The figure shows three views and two pictorial views of one solid part (mm, origin at its lowest corner). Answer the questions. A direction names the side the tool comes from. Coordinates: 2 decimals unless noted, no trailing zeros. Order: outer loops, then holes, each group sorted by start corner. A loop starts at its lowest first (then second) coordinate and runs counter-clockwise, first axis right, second up. Notation, with made-up numbers: (-6, 34.5) - (52, 34.5) arc R23 cw to (52, 70.5) - close; hole circle Ø4 at (-10.75, 74). An arc over 180 degrees is marked (long way). Answer as a JSON object with one key per item and string values. Group by question number.
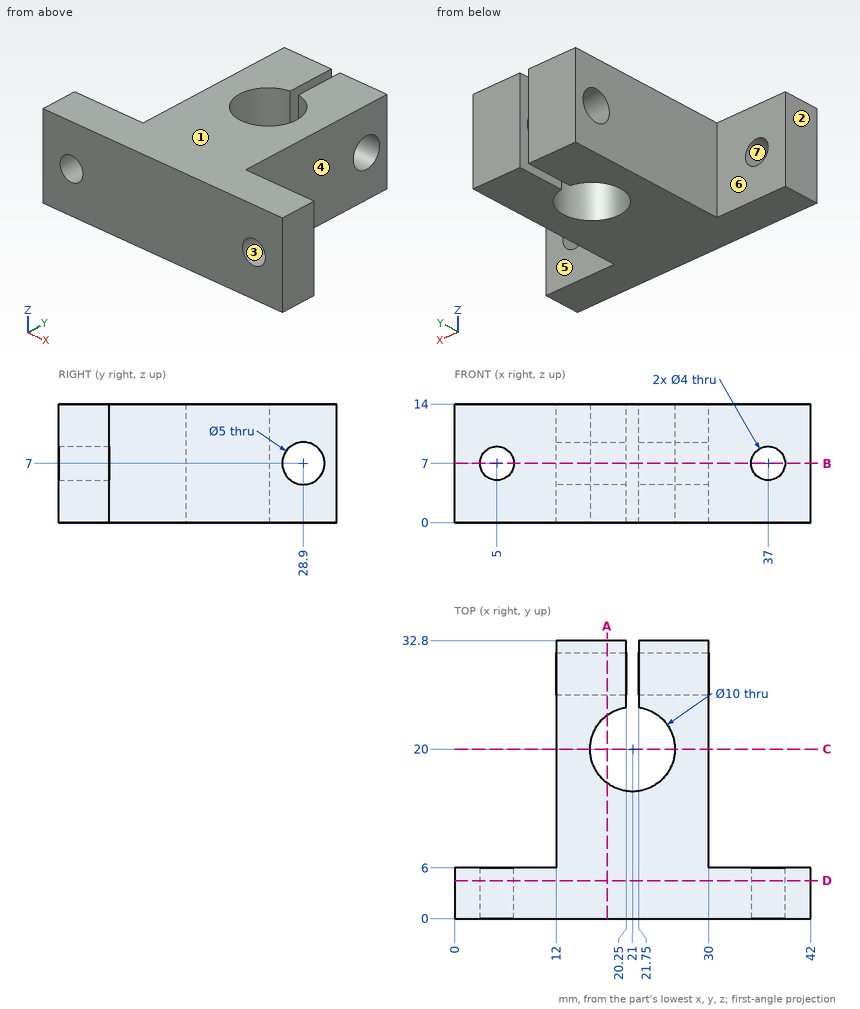
1. A cutting plane is placed at B-B on z = 7. Write down the section's boundary in (x, y).
2. A cutting plane is placed at A-A on x = 18. Write down the section's boundary in (y, z).
3. For a pull along X with two mould halves and no side action, classify the marked faces 1, 2, 3 and 4 as pulls with the +X half, pulls with the -X half, needs draft (parallel to the pull), parting line crosses it, or undercut.
4. Given pin 1 (4 mm diameter, centred on y = 30.5, z = 5.5, fed in from +X); pin 2 (3 mm diameter, centred on y = 16.5, z = 11.5, fed in from -X); pin 3 (3.5 mm diameter, centred on x = 6.5, z = 7.5, fed in from +Y); pin 4 (8 mm diameter, centred on y = 9.5, z = 9, fed in from -X), each flat-ended and moving along its own axis, determine where each tip first touches the part or whether it passes through.
5. For the marked faces 5, 6 and 7, determine the directions among +Z, -Z, +X, -X, +Y, -Y from which every point of the face is accessible in a straight line to the end or side of a thin tool.
6. Straight lines are drawn through the part: L1, parallel to X at y = 25, z = 3.25; L2, parallel to X at y = 20, z = 10; L3, parallel to Y at x = 20, z = 7.5. For each, find the intervals that lie inside material, in ascending order.
7. A cutting plane is placed at D-D on y = 4.5. Write down the section's boundary in (x, z).
8. A cutting plane is placed at C-C on y = 20. Write down the section's boundary in (x, z), and give its area (3 significant figures).
Derived:
{
 "1": {"outline": "(0, 0) - (3, 0) - (3, 6) - (0, 6) - close; (7, 0) - (35, 0) - (35, 6) - (30, 6) - (30, 26.4) - (21.75, 26.4) - (21.75, 24.94) arc R5 cw (long way) to (20.25, 24.94) - (20.25, 26.4) - (12, 26.4) - (12, 6) - (7, 6) - close; (12, 31.4) - (20.25, 31.4) - (20.25, 32.8) - (12, 32.8) - close; (21.75, 31.4) - (30, 31.4) - (30, 32.8) - (21.75, 32.8) - close; (39, 0) - (42, 0) - (42, 6) - (39, 6) - close"},
 "2": {"outline": "(0, 0) - (16, 0) - (16, 14) - (0, 14) - close; (24, 0) - (32.8, 0) - (32.8, 14) - (24, 14) - close; hole circle Ø5 at (28.9, 7)"},
 "3": {"face 1": "needs draft", "face 2": "pulls with the -X half", "face 3": "undercut", "face 4": "pulls with the +X half"},
 "4": {"pin 1": "stops at x = 30", "pin 2": "stops at x = 12", "pin 3": "stops at y = 6", "pin 4": "stops at x = 0"},
 "5": {"face 5": "+Z, -Z, +X, +Y", "face 6": "+Z, -Z, -X, +Y", "face 7": "+Y, -Y"},
 "6": {"L1": "x = 12 to 20.25, 21.75 to 30", "L2": "x = 12 to 16, 26 to 30", "L3": "y = 0 to 15.1, 24.9 to 26.45, 31.35 to 32.8"},
 "7": {"outline": "(0, 0) - (42, 0) - (42, 14) - (0, 14) - close; hole circle Ø4 at (5, 7); hole circle Ø4 at (37, 7)"},
 "8": {"outline": "(12, 0) - (16, 0) - (16, 14) - (12, 14) - close; (26, 0) - (30, 0) - (30, 14) - (26, 14) - close", "area": "112 mm2"}
}
